Read the model definition and answer for the solid it produces. Units are mm, in the model's axes. A direction names the side the tool comes from. Round coordinates to 2 decimals unless told otherwise and drop trailing zeros. Loops run counter-clockwise (first coordinate to the right, second up) from the corner with the lowest first, then second, coordinate; pieces in that order, holes last. Notation, with made-up numbers: M 41,-34 L 67,-34 A12 ccw 67,-29 Z; hole C 23,15.25 d5. An arc over 180 degrees is marked long. Write each question's results on one line, items separated by ' | '.
```python
from build123d import *

# Parameters (mm, degrees)
SKETCH1_W           = 61
SKETCH1_H           = 61
SKETCH1_W_2         = 55
SKETCH1_H_2         = 55
BOSS_EXTRUDE1_DEPTH = 60
SKETCH2_W           = 61
SKETCH2_H           = 61
BOSS_EXTRUDE2_DEPTH = 3
CUT_EXTRUDE1_DEPTH  = 3


with BuildPart() as part:
    # Sketch1 → Boss-Extrude1 (new body)
    with BuildSketch(Plane.XY):
        Rectangle(SKETCH1_W, SKETCH1_H)
        Rectangle(SKETCH1_W_2, SKETCH1_H_2, mode=Mode.SUBTRACT)
    extrude(amount=BOSS_EXTRUDE1_DEPTH)

    # Sketch2 → Boss-Extrude2 (add)
    with BuildSketch(Plane(origin=(0, 0, 0), x_dir=(-1, 0, 0), z_dir=(0, 0, -1))):
        Rectangle(SKETCH2_W, SKETCH2_H)
    extrude(amount=-BOSS_EXTRUDE2_DEPTH)

    # Sketch3 → Cut-Extrude1 (cut)
    with BuildSketch(Plane(origin=(0, 0, 0), x_dir=(-1, 0, 0), z_dir=(0, 0, -1))):
        with BuildLine():
            ThreePointArc((14, -9.5), (12.939339828, -9.939339828), (12.5, -11))
            Line((12.5, -11), (14, -11))
            Line((14, -11), (14, -9.5))
        make_face()
        with BuildLine():
            Line((14, -11), (12.5, -11))
            ThreePointArc((12.5, -11), (14, -12.5), (15.5, -11))
            ThreePointArc((15.5, -11), (15.060660172, -9.939339828), (14, -9.5))
            Line((14, -9.5), (14, -11))
        make_face()
        with BuildLine():
            Line((-14, -9.5), (-14, -11))
            Line((-14, -11), (-12.5, -11))
            ThreePointArc((-12.5, -11), (-12.939339828, -9.939339828), (-14, -9.5))
        make_face()
        with BuildLine():
            Line((-12.5, -11), (-14, -11))
            Line((-14, -11), (-14, -9.5))
            ThreePointArc((-14, -9.5), (-15.060660172, -12.060660172), (-12.5, -11))
        make_face()
        with BuildLine():
            ThreePointArc((12.5, 11), (12.939339828, 9.939339828), (14, 9.5))
            Line((14, 9.5), (14, 11))
            Line((14, 11), (12.5, 11))
        make_face()
        with BuildLine():
            Line((14, 11), (14, 9.5))
            ThreePointArc((14, 9.5), (15.060660172, 9.939339828), (15.5, 11))
            ThreePointArc((15.5, 11), (14, 12.5), (12.5, 11))
            Line((12.5, 11), (14, 11))
        make_face()
        with BuildLine():
            ThreePointArc((-12.5, 11), (-15.060660172, 12.060660172), (-14, 9.5))
            Line((-14, 9.5), (-14, 11))
            Line((-14, 11), (-12.5, 11))
        make_face()
        with BuildLine():
            Line((-14, 11), (-14, 9.5))
            ThreePointArc((-14, 9.5), (-12.939339828, 9.939339828), (-12.5, 11))
            Line((-12.5, 11), (-14, 11))
        make_face()
    extrude(amount=-CUT_EXTRUDE1_DEPTH, mode=Mode.SUBTRACT)


solid = part.part
```
1. Determine the mould class of faces 1 (the face through (27.5, 0, 31)), 2 (the face through (-27.5, 0, 31)), 3 (the face through (0, -30.5, 30)), 4 (the face through (0, 0, 0)) for opening direction Y: released by +Y, released by -Y, zero draft, split by the parting line, or undercut.
Completed:
face 1: undercut | face 2: undercut | face 3: released by -Y | face 4: zero draft
2. Given P1, Ø1, axis at x = -3.5, y = -3.5, coming from the +Z side, flat-ended and moving along its own axis, determine where the tip first touches the part or whether it passes through.
Completed:
P1: stops at z = 3
3. Which of the six approach directions +Z, -Z, +X, -X, +Y, -Y give full straight-line access (tool end or side, diameter ignored) to faces 5 (the face through (0, 27.5, 31)), 6 (the face through (0, 30.5, 30))?
Completed:
face 5: +Z | face 6: +Z, -Z, +X, -X, +Y
4. Find section A-A, the plane y = -18.5. Give the vertices of the cut face in (x, z).
Completed:
outline: M -30.5,0 L 30.5,0 L 30.5,60 L 27.5,60 L 27.5,3 L -27.5,3 L -27.5,60 L -30.5,60 Z
5. Find section B-B, the plane z = 9. Give the vertices of the cut face in (x, y).
Completed:
outline: M -30.5,-30.5 L 30.5,-30.5 L 30.5,30.5 L -30.5,30.5 Z; hole M -27.5,-27.5 L 27.5,-27.5 L 27.5,27.5 L -27.5,27.5 Z
6. Find the intervals of material crossed by L1, parallel to Y at x = 14, z = 1.7; L2, parallel to X at y = -11, z = 0.8; L3, parallel to Y at x = 6, z = 24.5, in increasing order.
Completed:
L1: y = -30.5 to -12.5, -9.5 to 9.5, 12.5 to 30.5 | L2: x = -30.5 to -15.5, -12.5 to 12.5, 15.5 to 30.5 | L3: y = -30.5 to -27.5, 27.5 to 30.5
